from build123d import *
from OCP.BRepFilletAPI import BRepFilletAPI_MakeChamfer

# Parameters (mm, degrees)
SKETCH1_R           = 25.4
BOSS_EXTRUDE1_DEPTH = 279.4
SKETCH2_R           = 31.75
BOSS_EXTRUDE2_DEPTH = 25.4
CUT_EXTRUDE1_DEPTH  = 12.7
FILLET1_R           = 2.54
CHAMFER1_SIZE       = 2.54
CHAMFER1_SIZE2      = 8.858032687


with BuildPart() as part:
    # Sketch1 → Boss-Extrude1 (new body)
    with BuildSketch(Plane(origin=(0, 0, 0), x_dir=(1, 0, 0), z_dir=(0, 1, 0))):
        with Locations(Location((0, 0, 0), (0, 0, 270))):
            Circle(SKETCH1_R)
    extrude(amount=BOSS_EXTRUDE1_DEPTH)

    # Sketch2 → Boss-Extrude2 (add)
    with BuildSketch(Plane.XZ):
        with Locations(Location((0, 0, 0), (0, 0, 270))):
            Circle(SKETCH2_R)
    extrude(amount=BOSS_EXTRUDE2_DEPTH)

    # Sketch3 → Cut-Extrude1 (cut)
    with BuildSketch(Plane.XZ.offset(25.4)):
        Polygon((25.303831814, 0), (17.892511066, 17.892511066), (0, 25.303831814), (-17.892511066, 17.892511066), (-25.303831814, 0), (-17.892511066, -17.892511066), (0, -25.303831814), (17.892511066, -17.892511066), align=None)
    extrude(amount=-CUT_EXTRUDE1_DEPTH, mode=Mode.SUBTRACT)

    # Fillet1
    fillet1_edges = [part.edges().sort_by_distance(p)[0] for p in [
        (0, -25.4, 31.75),
    ]]
    fillet(fillet1_edges, radius=FILLET1_R)

    # Chamfer1: one chamfer whose edges measure the first distance from different faces: ONE call of the kernel's chamfer builder (chamfer() names one face for all edges)
    chamfer1_edges_1 = [part.edges().sort_by_distance(p)[0] for p in [
        (8.946255533, -12.7, 21.59817144),
    ]]
    chamfer1_side_1 = [part.faces().sort_by_distance(p)[0] for p in [
        (8.946255533, -19.05, 21.59817144),
    ]]
    chamfer1_edges_2 = [part.edges().sort_by_distance(p)[0] for p in [
        (21.59817144, -12.7, 8.946255533),
    ]]
    chamfer1_side_2 = [part.faces().sort_by_distance(p)[0] for p in [
        (21.59817144, -19.05, 8.946255533),
    ]]
    chamfer1_edges_3 = [part.edges().sort_by_distance(p)[0] for p in [
        (21.59817144, -12.7, -8.946255533),
    ]]
    chamfer1_side_3 = [part.faces().sort_by_distance(p)[0] for p in [
        (21.59817144, -19.05, -8.946255533),
    ]]
    chamfer1_edges_4 = [part.edges().sort_by_distance(p)[0] for p in [
        (8.946255533, -12.7, -21.59817144),
    ]]
    chamfer1_side_4 = [part.faces().sort_by_distance(p)[0] for p in [
        (8.946255533, -19.05, -21.59817144),
    ]]
    chamfer1_edges_5 = [part.edges().sort_by_distance(p)[0] for p in [
        (-8.946255533, -12.7, -21.59817144),
    ]]
    chamfer1_side_5 = [part.faces().sort_by_distance(p)[0] for p in [
        (-8.946255533, -19.05, -21.59817144),
    ]]
    chamfer1_edges_6 = [part.edges().sort_by_distance(p)[0] for p in [
        (-21.59817144, -12.7, -8.946255533),
    ]]
    chamfer1_side_6 = [part.faces().sort_by_distance(p)[0] for p in [
        (-21.59817144, -19.05, -8.946255533),
    ]]
    chamfer1_edges_7 = [part.edges().sort_by_distance(p)[0] for p in [
        (-21.59817144, -12.7, 8.946255533),
    ]]
    chamfer1_side_7 = [part.faces().sort_by_distance(p)[0] for p in [
        (-21.59817144, -19.05, 8.946255533),
    ]]
    chamfer1_edges_8 = [part.edges().sort_by_distance(p)[0] for p in [
        (-8.946255533, -12.7, 21.59817144),
    ]]
    chamfer1_side_8 = [part.faces().sort_by_distance(p)[0] for p in [
        (-8.946255533, -19.05, 21.59817144),
    ]]
    chamfer1 = BRepFilletAPI_MakeChamfer(part.part.solid().wrapped)
    for e in chamfer1_edges_1:
        chamfer1.Add(CHAMFER1_SIZE, CHAMFER1_SIZE2, e.wrapped, chamfer1_side_1[0].wrapped)  # the first distance lies on this face
    for e in chamfer1_edges_2:
        chamfer1.Add(CHAMFER1_SIZE, CHAMFER1_SIZE2, e.wrapped, chamfer1_side_2[0].wrapped)  # the first distance lies on this face
    for e in chamfer1_edges_3:
        chamfer1.Add(CHAMFER1_SIZE, CHAMFER1_SIZE2, e.wrapped, chamfer1_side_3[0].wrapped)  # the first distance lies on this face
    for e in chamfer1_edges_4:
        chamfer1.Add(CHAMFER1_SIZE, CHAMFER1_SIZE2, e.wrapped, chamfer1_side_4[0].wrapped)  # the first distance lies on this face
    for e in chamfer1_edges_5:
        chamfer1.Add(CHAMFER1_SIZE, CHAMFER1_SIZE2, e.wrapped, chamfer1_side_5[0].wrapped)  # the first distance lies on this face
    for e in chamfer1_edges_6:
        chamfer1.Add(CHAMFER1_SIZE, CHAMFER1_SIZE2, e.wrapped, chamfer1_side_6[0].wrapped)  # the first distance lies on this face
    for e in chamfer1_edges_7:
        chamfer1.Add(CHAMFER1_SIZE, CHAMFER1_SIZE2, e.wrapped, chamfer1_side_7[0].wrapped)  # the first distance lies on this face
    for e in chamfer1_edges_8:
        chamfer1.Add(CHAMFER1_SIZE, CHAMFER1_SIZE2, e.wrapped, chamfer1_side_8[0].wrapped)  # the first distance lies on this face
    add(Compound.cast(chamfer1.Shape()), mode=Mode.REPLACE)


solid = part.part
Verification items for the finished model (mm, model axes). A direction names the side the tool comes from. Give positions to 0.01 mm unless a question says otherwise; leave off trailing zeros. Loops run counter-clockwise (first coordinate to the right, second up) from the corner with the lowest first, then second, coordinate; pieces in that order, holes last.
1) Set-up check for faces 1 (the flat face through (21.3, 0, 14.3)), 2 (the flat face through (-21.65, -20.39, -8.82)): record each of +Z, -Z, +X, -X, +Y, -Y from which the full face is reachable in a straight line by a thin tool's end or side.
2) Thickness scan on line 1 along Y through (x, z) = (-4, -10.5); line 2 along Z through (x, y) = (18, 164); line 3 along Z through (x, y) = (1.5, 71.5). Record the ranges inside material, lowest first.
3) Sectioned sample at A-A, the plane y = 116.5. Enter the section's corners in (x, z), then the cut area to 3 significant figures.
4) Draft check along X on faces 3 (the flat face through (-22, -25.4, -11)), 4 (the cylindrical face through (-15.456, 137.744, -20.157)), 5 (the flat face through (9.072, -20.391, 21.546)). Enter one of: pulls with the +X half, pulls with the -X half, needs draft (parallel to the pull), parting line crosses it, or undercut.
5) Depth check by flat-ended pin: pin 1 Ø10 at (x, y) = (21.5, 149) entering from +Z; pin 2 Ø2 at (y, z) = (82.5, 7.5) entering from +X; pin 3 Ø6 at (y, z) = (156, -2.5) entering from -X. Enter the tip coordinate at first touch or a pass-through.
Answers:
1. face 1: +Y
1. face 2: -Y
2. line 1: y = -12.7 to 279.4
2. line 2: z = -17.92 to 17.92
2. line 3: z = -25.36 to 25.36
3. outline: circle Ø50.8 at (0, 0)
3. area: 2,030 mm2
4. face 3: needs draft
4. face 4: parting line crosses it
4. face 5: undercut
5. pin 1: stops at z = 19.31
5. pin 2: stops at x = 24.55
5. pin 3: stops at x = -25.4
